Check sheet for the drawn part. Datum: minimum x, y, z corner. Units: mm. A direction names the side the tool comes from. Give positions to 0.01 mm unless a question says otherwise; leave off trailing zeros. Order: outer loops, then holes, each group sorted by start corner. A loop starts at its lowest first (then second) coordinate and runs counter-clockwise, first axis right, second up. Notation, with made-up numbers: (47.25, 78.25) -> (71.25, 78.25) arc R36 ccw to (71.25, 112.25) -> close; hole circle Ø6 at (47, 53.25). An arc over 180 degrees is marked (long way). Return JSON: item names as keys, results as strings. Group by question number.
(1) Depth check by flat-ended pin: pin 1 Ø2.5 at (x, y) = (12.5, 21) entering from -Z; pin 2 Ø1 at (x, y) = (19, 16.5) entering from +Z; pin 3 Ø1.5 at (x, y) = (13, 4) entering from +Z; pin 4 Ø2 at (y, z) = (12, 43.5) entering from -X. Enter the tip coordinate at first touch or a pass-through.
(2) Tool access check on the marked faces 1 and 2. Record the directions out of +Z, -Z, +X, -X, +Y, -Y that give a thin tool (end or side, any length) a straight path to the whole face; none if there is none.
(3) Cross-section at A-A on x = 12.5. Enter the section's corners in (y, z).
(4) Cross-section at B-B on y = 12.5. Enter the section's corners in (x, z).
(5) Thickness scan on line 1 along Y through (x, z) = (12.5, 34); line 2 along Y through (x, z) = (12.25, 23); line 3 along Z through (x, y) = (15.25, 13.75). Record the ranges inside material, lowest first.
(6) Cross-section at D-D on y = 4. Enter the section's corners in (x, z).
(7) Cross-section at C-C on z = 24. Enter the section's corners in (x, y), then the cut area to 3 significant figures.
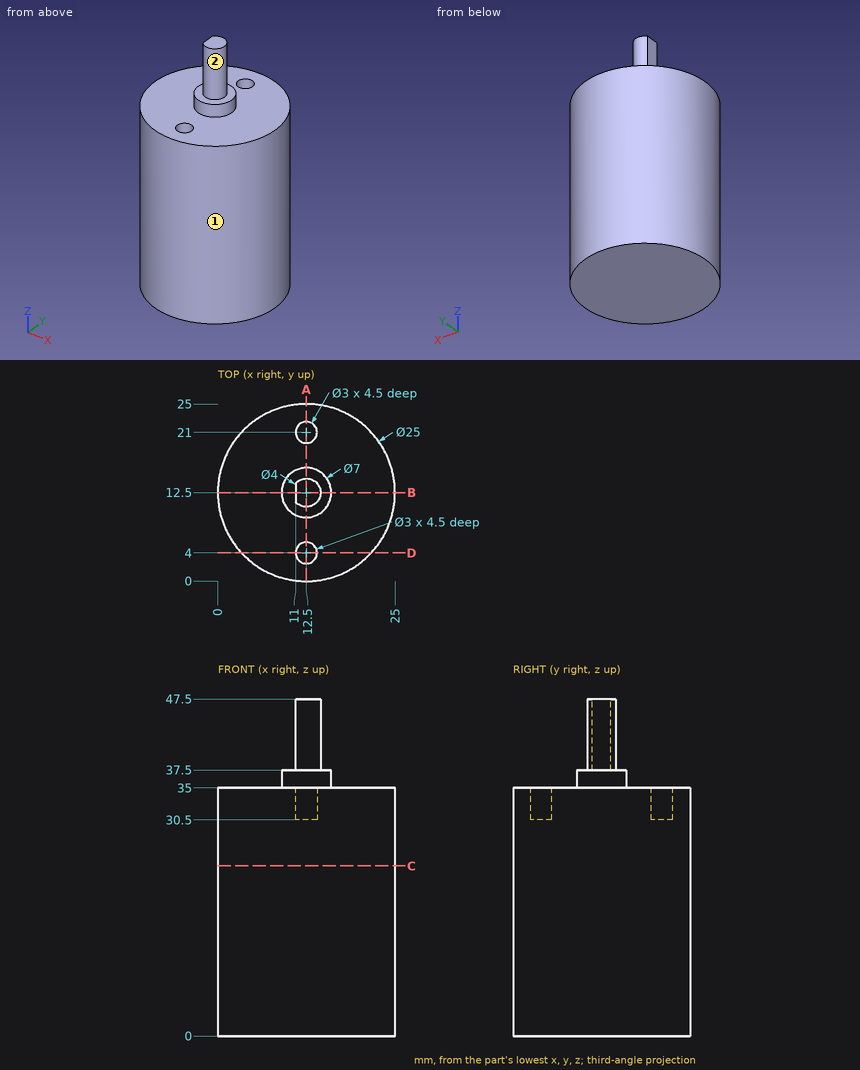
Verdict:
{
 "1": {"pin 1": "z = 0", "pin 2": "z = 35", "pin 3": "z = 30.5", "pin 4": "x = 11"},
 "2": {"face 1": "+Z, -Z", "face 2": "+Z"},
 "3": {"outline": "(0, 0) -> (25, 0) -> (25, 35) -> (22.5, 35) -> (22.5, 30.5) -> (19.5, 30.5) -> (19.5, 35) -> (16, 35) -> (16, 37.5) -> (14.5, 37.5) -> (14.5, 47.5) -> (10.5, 47.5) -> (10.5, 37.5) -> (9, 37.5) -> (9, 35) -> (5.5, 35) -> (5.5, 30.5) -> (2.5, 30.5) -> (2.5, 35) -> (0, 35) -> close"},
 "4": {"outline": "(0, 0) -> (25, 0) -> (25, 35) -> (16, 35) -> (16, 37.5) -> (14.5, 37.5) -> (14.5, 47.5) -> (11, 47.5) -> (11, 37.5) -> (9, 37.5) -> (9, 35) -> (0, 35) -> close"},
 "5": {"line 1": "0 to 2.5, 5.5 to 19.5, 22.5 to 25", "line 2": "0 to 25", "line 3": "0 to 37.5"},
 "6": {"outline": "(3.33, 0) -> (21.67, 0) -> (21.67, 35) -> (14, 35) -> (14, 30.5) -> (11, 30.5) -> (11, 35) -> (3.33, 35) -> close"},
 "7": {"outline": "circle Ø25 at (12.5, 12.5)", "area": "491 mm²"}
}
